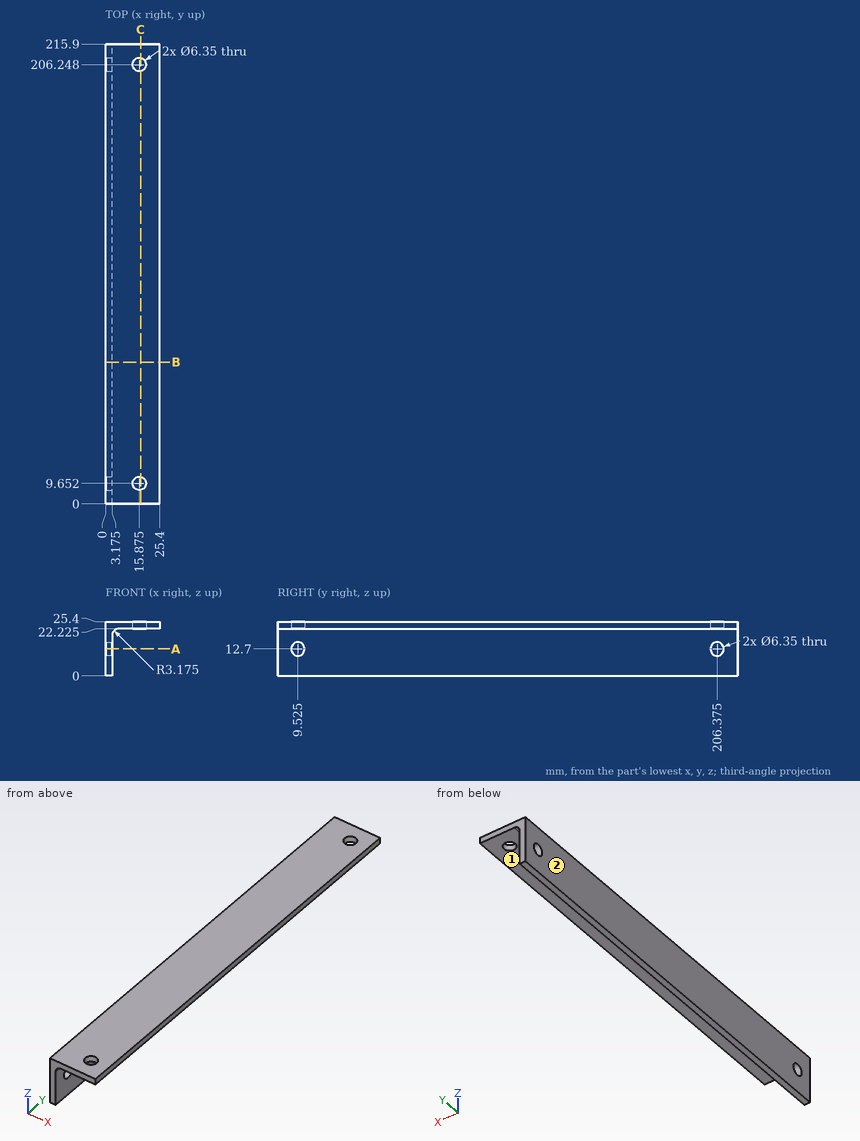
Geometry: see drawing. Coordinates: mm, zero at the bounding-box minimum. A direction names the side the tool comes from. Give positions to 0.01 mm unless a question says otherwise; leave off trailing zeros. Write each loop counter-clockwise with the first axis right and the second up, starting at its lowest first coordinate (ties: lowest second). Pieces come first, ordered by that corner, then holes. Notation, with made-up numbers: M -35,49 L 5,49 A22 cw 5,83 Z; hole C 35,37 d1. An arc over 180 degrees is marked long. Return JSON: item names as keys, results as strings. Group by question number.
1) Cut plane B-B, the plane y = 66.5. Output: boundary loops of the cut face in (x, z) (3 decimals).
2) Cut plane A-A, the plane z = 12.7. Output: boundary loops of the cut face in (x, y) (3 decimals), then the cut area to 3 significant figures.
3) Set-up query: the marked faces 1 and 2. Return all of +Z, -Z, +X, -X, +Y, -Y with unobstructed straight access to the full face (end or side cutting, diameter ignored); none if empty.
4) Cut plane C-C, the plane x = 16.5. Output: boundary loops of the cut face in (y, z) (3 decimals), then the cut area to 3 significant figures.
5) Ray query, L1, parallel to Y at x = 1.35, z = 12.7; L2, parallel to Z at x = 6.25, y = 116.5; L3, parallel to X at y = 43.5, z = 5 (3 decimals). Return the intervals inside material, ascending.
6) First-contact query: pin 1 Ø8 at (y, z) = (65.5, 15.5) entering from +X; pin 2 Ø1.5 at (y, z) = (170.5, 21.5) entering from -X; pin 3 Ø7.5 at (x, y) = (15.875, 9.652) entering from -Z (3 decimals). Flat tips, straight axial feed; report the tip coordinate or a pass-through.
Data:
{
 "1": {"outline": "M 0,0 L 3.175,0 L 3.175,19.05 A3.175 cw 6.35,22.225 L 25.4,22.225 L 25.4,25.4 L 0,25.4 Z"},
 "2": {"outline": "M 0,0 L 3.175,0 L 3.175,6.35 L 0,6.35 Z; M 0,12.7 L 3.175,12.7 L 3.175,203.2 L 0,203.2 Z; M 0,209.55 L 3.175,209.55 L 3.175,215.9 L 0,215.9 Z", "area": "645 mm²"},
 "3": {"face 1": "-Z, +X, +Y, -Y", "face 2": "+Z, -Z, -X, +Y, -Y"},
 "4": {"outline": "M 0,22.225 L 6.539,22.225 L 6.539,25.4 L 0,25.4 Z; M 12.765,22.225 L 203.135,22.225 L 203.135,25.4 L 12.765,25.4 Z; M 209.361,22.225 L 215.9,22.225 L 215.9,25.4 L 209.361,25.4 Z", "area": "646 mm²"},
 "5": {"L1": "y = 0 to 6.35, 12.7 to 203.2, 209.55 to 215.9", "L2": "z = 22.22 to 25.4", "L3": "x = 0 to 3.175"},
 "6": {"pin 1": "stops at x = 3.21", "pin 2": "stops at x = 0", "pin 3": "stops at z = 22.225"}
}
